Autodesk Inventor part; units mm, degrees
ref_plane "YZ Plane" through (0, 0, 0) normal (1, 0, 0) x (0, 1, 0)
ref_plane "XZ Plane" through (0, 0, 0) normal (0, 1, 0) x (-1, 0, 0)
ref_plane "XY Plane" through (0, 0, 0) normal (0, 0, 1) x (1, 0, 0)
sketch "Sketch1" plane through (0, 0, 0) normal (0, 1, 0) x (-1, 0, 0)
  line L0 (-7.5, -30) -> (7.5, -30)
  line L1 (7.5, -30) -> (7.5, 30)
  line L2 (7.5, 30) -> (-7.5, 30)
  line L3 (-7.5, 30) -> (-7.5, -30)
  line L4 (-7.5, -30) -> (7.5, 30) construction
  line L5 (7.5, -30) -> (-7.5, 30) construction
  point P0 (0, 0)
  dimension "d0" = 15
  dimension "d1" = 60
extrude "Extrusion1" add sketch "Sketch1" along normal blind 3
sketch "Sketch2" plane through (0, 3, 0) normal (0, 1, 0) x (1, 0, 0)
  line L0 (-7.5, 30) -> (-7.5, -30)
  line L1 (7.5, 20.5) -> (-7.5, 20.5)
  line L2 (-7.5, 20.5) -> (-7.5, -20.5)
  line L3 (-7.5, -20.5) -> (7.5, -20.5)
  line L4 (7.5, -20.5) -> (7.5, 20.5)
  line L5 (7.5, 20.5) -> (-7.5, -20.5) construction
  line L6 (-7.5, 20.5) -> (7.5, -20.5) construction
  line L7 (7.5, -20.5) -> (-7.5, -20.5)
  line L8 (-7.5, -20.5) -> (-7.5, -30)
  line L9 (-7.5, -30) -> (7.5, -30)
  line L10 (7.5, -30) -> (7.5, -20.5)
  line L11 (7.5, 30) -> (-7.5, 30)
  line L12 (7.5, 20.5) -> (-7.5, 20.5)
  line L13 (-7.5, 20.5) -> (-7.5, 30)
  line L14 (-7.5, 30) -> (7.5, 30)
  line L15 (7.5, 30) -> (7.5, 20.5)
  point P0 (0, 0)
  dimension "d4" = 41
extrude "Extrusion2" add sketch "Sketch2" along normal blind 19 contours L11 L15 L1 L0 | L3 L10 L9 L0
sketch "Sketch3" plane through (-7.5, 0, -30) normal (-1, 0, 0) x (0, 0, 1)
  line L0 (60, 0) -> (0, 0)
  line L1 (60, 0) -> (50, 0)
  line L2 (50, 0) -> (50, -21.64)
  line L3 (50, -21.64) -> (60, -21.64)
  line L4 (60, -21.64) -> (60, 0)
  point P0 (30, 0)
  dimension "d7" = 10
  dimension "d8" = 21.64
extrude "Extrusion3" add sketch "Sketch3" against normal blind 15
sketch "Sketch5" plane through (-7.5, 0, -30) normal (-1, 0, 0) x (0, 0, 1)
  line L0 (0, 0) -> (50, 0)
  line L1 (28.3595, 0) -> (50, -21.6405)
  line L2 (50, -21.64) -> (50, 0)
  line L3 (28.3595, 0) -> (58.9638, 0) construction
  line L4 (50, -21.6405) -> (50, 0)
  line L5 (50, 0) -> (28.3595, 0)
  point P0 (30, 0)
  dimension "d15" = 45
extrude "Extrusion5" add sketch "Sketch5" against normal blind 15
sketch "Sketch6" plane through (-7.5, 0, -30) normal (-1, 0, 0) x (0, 0, 1)
  line L0 (60, -21.64) -> (60, 22)
  line L1 (60, -21.64) -> (50.1294, -21.64)
  line L2 (50.1294, -21.64) -> (50.1294, -11.769)
  line L3 (50.1294, -11.769) -> (60, -11.769)
  line L4 (60, -11.769) -> (60, -21.64)
  point P0 (30, 0)
  dimension "d18" = 9.871
extrude "Extrusion6" add sketch "Sketch6" along normal blind 50
sketch "Sketch7" plane through (-7.5, 22, 30) normal (0, 0, 1) x (1, 0, 0)
  point P0 (7.5, -22)
fillet "Fillet1" radius 5 2 edges at (-57.5, -21.64, 25.0647) (-57.5, -11.769, 25.0647)
sketch "Sketch8" plane through (-7.5, -21.64, 20.1294) normal (0, 0, -1) x (-1, 0, 0)
  arc A0 (45, 0) -> (50, 5) centre (45, 5) ccw
  point P0 (-7.5, 21.64)
hole "Hole1" at (-52.5, -16.64, 20.1294) direction (0, 0, 1) diameter 3 end through all
properties part number "TurretServoSupport" material "PC/ABS Plastic"
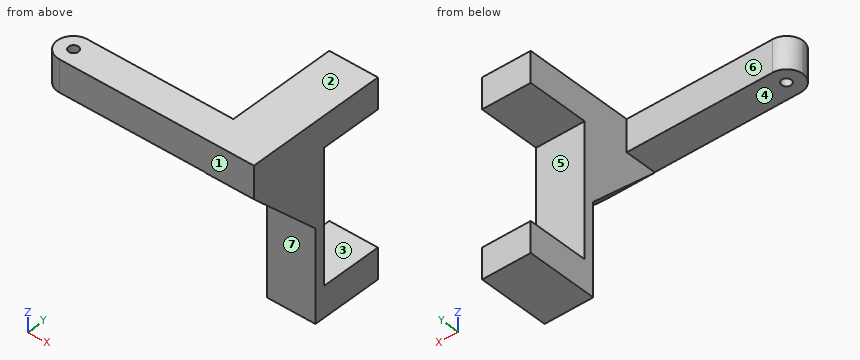
Verification items for the finished model (mm, model axes). Face numbers are marked on the shaded views. A direction names the side the tool comes from. Coordinates: 2 decimals unless noted, no trailing zeros. Write each loop counter-clockwise with the first axis right and the second up, starting at its lowest first coordinate (ties: lowest second). Pieces come first, ordered by that corner, then holes. Notation, with made-up numbers: (88.5, 87.25) - (127.5, 87.25) arc R16 cw to (127.5, 117.25) - close; hole circle Ø2 at (63.25, 19.25). An arc over 180 degrees is marked (long way). One line per question, with ' | ' between items. Start each with the question number.
1. Section check A-A (y = 14.5). Enter the section's corners in (x, z).
2. Access from +Z, -Z, +X, -X, +Y, -Y to the whole of each face (thin tool, end or side, straight path). Record for the marked faces 5, 6 and 7.
3. Draft check along Z on the marked faces 1, 2, 3 and 4. Enter one of: released by +Z, released by -Z, zero draft, split by the parting line, or undercut.
4. Gauge pin test, flat ends, axial feed: P1, Ø1, axis at x = 0, z = -19, coming from the -Y side; P2, Ø11, axis at x = -25.5, z = 24, coming from the +Y side; P3, Ø10, axis at x = 0, y = -7, coming from the -Z side. Record the tip position at first contact, or that the pin passes through.
5. Section check D-D (z = -19). Enter the section's corners in (x, y).
6. Section check B-B (z = 25). Enter the section's corners in (x, y).
7. Material ranges on line 1 along Y through (x, z) = (-52.5, 27.25); line 2 along X through (y, z) = (-16.64, 24); line 3 along Z through (x, y) = (-3, 16.5), recorded low to high.
Computed values:
1) outline: (-7.5, -30) - (7.5, -30) - (7.5, -20.5) - (-7.5, -20.5) - close; (-7.5, 20.5) - (7.5, 20.5) - (7.5, 30) - (-7.5, 30) - close
2) face 5: +X, -X, +Y | face 6: +Z, -Z, -X, +Y | face 7: -Z, +X, -X, -Y
3) face 1: zero draft | face 2: released by +Z | face 3: undercut | face 4: released by -Z
4) P1: y = 0 | P2: y = -11.77 | P3: z = 0.36
5) outline: (-7.5, 0) - (7.5, 0) - (7.5, 3) - (-7.5, 3) - close
6) outline: (-57.5, -16.7) arc R5 ccw to (-52.5, -21.64) - (7.5, -21.64) - (7.5, 22) - (-7.5, 22) - (-7.5, -11.77) - (-52.5, -11.77) arc R5 ccw to start; hole circle Ø3 at (-52.5, -16.64)
7) line 1: -21.64 to -18.14, -15.14 to -11.77 | line 2: -57.5 to -54, -51 to 7.5 | line 3: -30 to -20.5, 20.5 to 30
